```python
from build123d import *

# Parameters (mm, degrees)
SKETCH1_R           = 13.8
BOSS_EXTRUDE1_DEPTH = 37.6
SKETCH2_R           = 5
BOSS_EXTRUDE2_DEPTH = 1.5
SKETCH3_R           = 1.15
BOSS_EXTRUDE3_DEPTH = 9.7
SKETCH4_R           = 1
CUT_EXTRUDE1_DEPTH  = 5
SKETCH5_R           = 5
BOSS_EXTRUDE4_DEPTH = 2.5
SKETCH6_W           = 0.5
SKETCH6_H           = 3
BOSS_EXTRUDE5_DEPTH = 7.5
SKETCH7_W           = 1.5
SKETCH7_H           = 2.5
CUT_EXTRUDE2_DEPTH  = 24.5
CHAMFER1_SIZE       = 0.5
FILLET1_R           = 0.5
SKETCH8_R           = 14.2
SKETCH8_R_2         = 13.8
BOSS_EXTRUDE6_DEPTH = 21


with BuildPart() as part:
    # Sketch1 → Boss-Extrude1 (new body)
    with BuildSketch(Plane(origin=(0, 0, 0), x_dir=(1, 0, 0), z_dir=(0, 1, 0))):
        Circle(SKETCH1_R)
    extrude(amount=BOSS_EXTRUDE1_DEPTH)

    # Sketch2 → Boss-Extrude2 (add)
    with BuildSketch(Plane(origin=(0, 37.6, 0), x_dir=(1, 0, 0), z_dir=(0, 1, 0))):
        Circle(SKETCH2_R)
    extrude(amount=BOSS_EXTRUDE2_DEPTH)

    # Sketch3 → Boss-Extrude3 (add)
    with BuildSketch(Plane(origin=(0, 39.1, 0), x_dir=(1, 0, 0), z_dir=(0, 1, 0))):
        Circle(SKETCH3_R)
    extrude(amount=BOSS_EXTRUDE3_DEPTH)

    # Sketch4 → Cut-Extrude1 (cut)
    with BuildSketch(Plane(origin=(0, 37.6, 0), x_dir=(1, 0, 0), z_dir=(0, 1, 0))):
        with Locations((8, 0)):
            Circle(SKETCH4_R)
        with Locations((-8, 0)):
            Circle(SKETCH4_R)
    extrude(amount=-CUT_EXTRUDE1_DEPTH, mode=Mode.SUBTRACT)

    # Sketch5 → Boss-Extrude4 (add)
    with BuildSketch(Plane.XZ):
        Circle(SKETCH5_R)
    extrude(amount=BOSS_EXTRUDE4_DEPTH)

    # Sketch6 → Boss-Extrude5 (add)
    with BuildSketch(Plane.XZ):
        with Locations((12, 0)):
            Rectangle(SKETCH6_W, SKETCH6_H)
        with Locations((-12, 0)):
            Rectangle(SKETCH6_W, SKETCH6_H)
    extrude(amount=BOSS_EXTRUDE5_DEPTH)

    # Sketch7 → Cut-Extrude2 (cut)
    with BuildSketch(Plane(origin=(12.25, 0, 0), x_dir=(0, 0, -1), z_dir=(1, 0, 0))):
        with Locations((0, -4.5)):
            Rectangle(SKETCH7_W, SKETCH7_H)
    extrude(amount=-CUT_EXTRUDE2_DEPTH, mode=Mode.SUBTRACT)

    # Chamfer1
    chamfer1_edges = [part.edges().sort_by_distance(p)[0] for p in [
        (12, -7.5, 1.5),
        (12, -7.5, -1.5),
        (-12, -7.5, 1.5),
        (-12, -7.5, -1.5),
    ]]
    chamfer(chamfer1_edges, length=CHAMFER1_SIZE)

    # Fillet1
    fillet1_edges = [part.edges().sort_by_distance(p)[0] for p in [
        (12, -3.25, -0.75),
        (-12, -3.25, -0.75),
        (12, -5.75, -0.75),
        (-12, -5.75, -0.75),
        (12, -5.75, 0.75),
        (-12, -5.75, 0.75),
        (12, -3.25, 0.75),
        (-12, -3.25, 0.75),
    ]]
    fillet(fillet1_edges, radius=FILLET1_R)

    # Sketch8 → Boss-Extrude6 (add)
    with BuildSketch(Plane(origin=(0, 33.6, 0), x_dir=(1, 0, 0), z_dir=(0, 1, 0))):
        Circle(SKETCH8_R)
        Circle(SKETCH8_R_2, mode=Mode.SUBTRACT)
    extrude(amount=-BOSS_EXTRUDE6_DEPTH)


solid = part.part
```
Work out the finished part from the listing and answer in its coordinate system (mm). A direction names the side the tool comes from. Give positions to 0.01 mm unless a question says otherwise; leave off trailing zeros. Loops run counter-clockwise (first coordinate to the right, second up) from the corner with the lowest first, then second, coordinate; pieces in that order, holes last. Notation, with made-up numbers: (-25.5, 54) -> (9.5, 54) arc R24 ccw to (9.5, 77) -> close; hole circle Ø10 at (80, 24.5). An arc over 180 degrees is marked (long way). Use CSV: the item, a comma, the result in double quotes.
1. Flat-ended cylindrical pins translate along their axes: pin 1 Ø4 at (x, y) = (-11, 41.5) entering from +Z; pin 2 Ø1 at (y, z) = (1.5, -9.5) entering from -X; pin 3 Ø0.6 at (x, y) = (-12, -3) entering from -Z; pin 4 Ø0.9 at (y, z) = (-3.5, -0.5) entering from +X. Find the tip coordinate at first contact, or state that the pin passes through.
Found:
pin 1,"through"
pin 2,"x = -10.46"
pin 3,"z = -1.5"
pin 4,"x = 12.25"
2. The part is cut by section A-A (x = 0). Write down the section's boundary in (y, z).
Found:
outline,"(-2.5, -5) -> (0, -5) -> (0, -13.8) -> (12.6, -13.8) -> (12.6, -14.2) -> (33.6, -14.2) -> (33.6, -13.8) -> (37.6, -13.8) -> (37.6, -5) -> (39.1, -5) -> (39.1, -1.15) -> (48.8, -1.15) -> (48.8, 1.15) -> (39.1, 1.15) -> (39.1, 5) -> (37.6, 5) -> (37.6, 13.8) -> (33.6, 13.8) -> (33.6, 14.2) -> (12.6, 14.2) -> (12.6, 13.8) -> (0, 13.8) -> (0, 5) -> (-2.5, 5) -> close"
3. A tool of negligible diameter and unlimited length cuts with its end or side. For faces 1 (the cylindrical face through (-0.91, 43.88, 0.7)), 2 (the cylindrical face through (-1.08, -1.23, -4.88)), 3 (the flat face through (0, -2.5, 0)), from which of +Z, -Z, +X, -X, +Y, -Y can it reach the whole face along a straight path? Write none if from no direction.
Found:
face 1,"+Y"
face 2,"-Y"
face 3,"+Z, -Z, -Y"
4. The part is cut by section B-B (z = 7.5). Write down the section's boundary in (x, y), then the cut area to 3 significant figures.
Found:
outline,"(-12.06, 12.6) -> (-11.58, 12.6) -> (-11.58, 0) -> (11.58, 0) -> (11.58, 12.6) -> (12.06, 12.6) -> (12.06, 33.6) -> (11.58, 33.6) -> (11.58, 37.6) -> (-11.58, 37.6) -> (-11.58, 33.6) -> (-12.06, 33.6) -> close"
area,"891 mm^2"
5. The mould has two halves that part along Z. Classify faces 4 (the cylindrical face through (-1.08, 38.34, 4.88)), 5 (the flat face through (-8, 32.6, 0)), 6 (the flat face through (-11.75, -3, 0)): +Z half, -Z half, draft (parallel to the pull), parting line (faces both ways), or undercut.
Found:
face 4,"parting line"
face 5,"undercut"
face 6,"draft"
6. The part is cut by section D-D (y = 36.5). Write down the section's boundary in (x, z).
Found:
outline,"circle Ø27.6 at (0, 0); hole circle Ø2 at (-8, 0); hole circle Ø2 at (8, 0)"
7. Straight lines are drawn through the part: line 1 (X direction, y = 36.45, z = 0); line 2 (Y direction, x = -0.25, z = -8.75); line 3 (Z direction, x = 8, y = 36.45). For each, find the intervals that lie inside material, in ascending order.
Found:
line 1,"-13.8 to -9, -7 to 7, 9 to 13.8"
line 2,"0 to 37.6"
line 3,"-11.24 to -1, 1 to 11.24"
8. The part is cut by section C-C (y = 7.5). Write down the section's boundary in (x, z).
Found:
outline,"circle Ø27.6 at (0, 0)"
